from build123d import *

# Parameters (mm, degrees)
BOSS_EXTRUDE1_DEPTH     = 2
CUT_EXTRUDE1_DEPTH      = 120.295393457
CUT_EXTRUDE1_DEPTH_BACK = 120.295393457
SKETCH2_R               = 2.5


with BuildPart() as part:
    # Sketch1 → Boss-Extrude1 (new body)
    with BuildSketch(Plane.XY):
        with BuildLine():
            Line((0, 0), (-38.1, 38.1))
            Line((-38.1, 38.1), (-93.98, 38.1))
            ThreePointArc((-93.98, 38.1), (-113.03, 19.05), (-93.98, 0))
            Line((-93.98, 0), (0, 0))
        make_face()
    extrude(amount=BOSS_EXTRUDE1_DEPTH)

    # Sketch2 → Cut-Extrude1 (cut, two sides: drawn at the far end of the back side and taken through both)
    with BuildSketch(Plane.XY.offset(2).offset(-CUT_EXTRUDE1_DEPTH_BACK)):
        with Locations((-53.1876, 8.89)):
            Circle(SKETCH2_R)
        with Locations((-21.311773075, 6.35)):
            Circle(SKETCH2_R)
        with Locations((-33.909, 25.4)):
            Circle(SKETCH2_R)
    extrude(amount=CUT_EXTRUDE1_DEPTH + CUT_EXTRUDE1_DEPTH_BACK, mode=Mode.SUBTRACT)


solid = part.part
Part model, mm, in its own coordinate system. Round coordinates to 2 decimals unless told otherwise and drop trailing zeros. Write each loop counter-clockwise with the first axis right and the second up, starting at its lowest first coordinate (ties: lowest second). Pieces come first, ordered by that corner, then holes. Notation, with made-up numbers: (49.5, 21) - (106.5, 21) arc R15 cw to (106.5, 37) - close; hole circle Ø8 at (-17, -18). An arc over 180 degrees is marked (long way). Use CSV: the item, a comma, the result in double quotes.
Item 1: Slice it at C-C, the plane y = 12.5. Write the cut outline in (x, z), then the cut area to 3 significant figures.
Results list:
outline,"(-111.87, 0) - (-12.5, 0) - (-12.5, 2) - (-111.87, 2) - close"
area,"199 mm²"
Item 2: Flat gauge pins, fed straight in: P1, Ø8, axis at x = -82.5, y = 20, coming from the -Z side; P2, Ø4, axis at x = -33.909, y = 25.4, coming from the -Z side. Where does each tip first touch, or does it go through?
Results list:
P1,"stops at z = 0"
P2,"passes through"
Item 3: Pull direction X, two halves, no side cores. Call faces 1 (the cylindrical face through (-35.75, 27.09, 0.99)), 2 (the flat face through (-70, 19, 0)), 3 (the cylindrical face through (-19.97, 8.46, 0.99)), 4 (the cylindrical face through (-113.025, 19.469, 0.986)): pulls with the +X half, pulls with the -X half, needs draft (parallel to the pull), parting line crosses it, or undercut.
Results list:
face 1,"undercut"
face 2,"needs draft"
face 3,"undercut"
face 4,"pulls with the -X half"
Item 4: Slice it at D-D, the plane x = -103.5. Write the cut outline in (y, z), then the cut area to 3 significant figures.
Results list:
outline,"(2.55, 0) - (35.55, 0) - (35.55, 2) - (2.55, 2) - close"
area,"66.0 mm²"
Item 5: Wall check: L1, parallel to X at y = 7, z = 1.2; L2, parallel to X at y = 8.5, z = 0.7; L3, parallel to Y at x = -52, z = 0.9. Give the ranges that are in metal, low to high.
Results list:
L1,"x = -108.73 to -54.82, -51.55 to -23.73, -18.9 to -7"
L2,"x = -109.84 to -55.66, -50.72 to -22.59, -20.04 to -8.5"
L3,"y = 0 to 6.69, 11.09 to 38.1"
Item 6: Slice it at B-B, the plane y = 25.4. Write the cut outline in (x, z), then the cut area to 3 significant figures.
Results list:
outline,"(-111.94, 0) - (-36.41, 0) - (-36.41, 2) - (-111.94, 2) - close; (-31.41, 0) - (-25.4, 0) - (-25.4, 2) - (-31.41, 2) - close"
area,"163 mm²"
Item 7: Slice it at A-A, the plane z = 1.5. Write the cut outline in (x, y), then the cut area to 3 significant figures.
Results list:
outline,"(-93.98, 0) - (0, 0) - (-38.1, 38.1) - (-93.98, 38.1) arc R19.05 ccw to start; hole circle Ø5 at (-53.19, 8.89); hole circle Ø5 at (-33.91, 25.4); hole circle Ø5 at (-21.31, 6.35)"
area,"3,370 mm²"
